from build123d import *

# Parameters (mm, degrees)
CROQUIS1_W                = 138
CROQUIS1_H                = 220
SALIENTE_EXTRUIR1_DEPTH   = 15
CORTAR_EXTRUIR1_DEPTH     = 76.5
CROQUIS3_R                = 4.25
CORTAR_EXTRUIR2_DEPTH     = 76.5
CROQUIS4_R                = 6.5
CORTAR_EXTRUIR3_DEPTH     = 8
CROQUIS5_W                = 12
CROQUIS5_H                = 220
CORTAR_EXTRUIR4_DEPTH     = 4
TALADRO_ROSCADO_M41_D     = 3.3
TALADRO_ROSCADO_M41_DEPTH = 8
TALADRO_ROSCADO_M41_TIP   = 0.991420021
CORTAR_EXTRUIR5_DEPTH     = 8
CHAFL_N1_SIZE             = 2


with BuildPart() as part:
    # Croquis1 → Saliente-Extruir1 (new body)
    with BuildSketch(Plane.XY):
        Rectangle(CROQUIS1_W, CROQUIS1_H)
    extrude(amount=SALIENTE_EXTRUIR1_DEPTH)

    # Croquis2 → Cortar-Extruir1 (cut)
    with BuildSketch(Plane.XY.offset(15)):
        with BuildLine():
            Line((-56, 122.891872251), (-56, 98))
            ThreePointArc((-56, 98), (-50, 92), (-44, 98))
            Line((-44, 98), (-44, 122.891872251))
            Line((-44, 122.891872251), (-56, 122.891872251))
        make_face()
        with BuildLine():
            Line((44, 116.909766475), (44, 98))
            ThreePointArc((44, 98), (50, 92), (56, 98))
            Line((56, 98), (56, 116.909766475))
            Line((56, 116.909766475), (44, 116.909766475))
        make_face()
        with BuildLine():
            Line((44, -98), (44, -115.830663504))
            Line((44, -115.830663504), (56, -115.830663504))
            Line((56, -115.830663504), (56, -98))
            ThreePointArc((56, -98), (50, -92), (44, -98))
        make_face()
        with BuildLine():
            Line((-56, -98), (-56, -115.886145335))
            Line((-56, -115.886145335), (-44, -115.886145335))
            Line((-44, -115.886145335), (-44, -98))
            ThreePointArc((-44, -98), (-50, -92), (-56, -98))
        make_face()
    extrude(amount=-CORTAR_EXTRUIR1_DEPTH, mode=Mode.SUBTRACT)

    # Croquis3 → Cortar-Extruir2 (cut)
    with BuildSketch(Plane.XY.offset(15)):
        with Locations((-61.5, 82.5)):
            Circle(CROQUIS3_R)
        with Locations((-61.5, 23.7)):
            Circle(CROQUIS3_R)
        with Locations((-61.5, -35.1)):
            Circle(CROQUIS3_R)
        with Locations((-34, -78.5)):
            Circle(CROQUIS3_R)
        with Locations((34, -78.5)):
            Circle(CROQUIS3_R)
        with Locations((61.5, -35.1)):
            Circle(CROQUIS3_R)
        with Locations((61.5, 23.7)):
            Circle(CROQUIS3_R)
        with Locations((61.5, 82.5)):
            Circle(CROQUIS3_R)
    extrude(amount=-CORTAR_EXTRUIR2_DEPTH, mode=Mode.SUBTRACT)

    # Croquis4 → Cortar-Extruir3 (cut)
    with BuildSketch(Plane.XY.offset(15)):
        with Locations((-61.5, 82.5)):
            Circle(CROQUIS4_R)
        with Locations((-61.5, 23.7)):
            Circle(CROQUIS4_R)
        with Locations((-61.5, -35.1)):
            Circle(CROQUIS4_R)
        with Locations((-34, -78.5)):
            Circle(CROQUIS4_R)
        with Locations((61.5, -35.1)):
            Circle(CROQUIS4_R)
        with Locations((61.5, 23.7)):
            Circle(CROQUIS4_R)
        with Locations((61.5, 82.5)):
            Circle(CROQUIS4_R)
        with Locations((34, -78.5)):
            Circle(CROQUIS4_R)
    extrude(amount=-CORTAR_EXTRUIR3_DEPTH, mode=Mode.SUBTRACT)

    # Croquis5 → Cortar-Extruir4 (cut)
    with BuildSketch(Plane.XY.offset(15)):
        Rectangle(CROQUIS5_W, CROQUIS5_H)
    extrude(amount=-CORTAR_EXTRUIR4_DEPTH, mode=Mode.SUBTRACT)

    # Taladro roscado M41
    with Locations(Plane.XY.offset(11)):
        with Locations((0, 104), (0, 76), (0, 14), (0, -14), (0, -76), (0, -104)):
            Hole(TALADRO_ROSCADO_M41_D / 2, depth=TALADRO_ROSCADO_M41_DEPTH)
            with Locations((0, 0, -(TALADRO_ROSCADO_M41_DEPTH + TALADRO_ROSCADO_M41_TIP / 2))):  # 118° drill point
                Cone(0, TALADRO_ROSCADO_M41_D / 2, TALADRO_ROSCADO_M41_TIP, mode=Mode.SUBTRACT)

    # Croquis8 → Cortar-Extruir5 (cut)
    with BuildSketch(Plane(origin=(0, 0, 0), x_dir=(-1, 0, 0), z_dir=(0, 0, -1))):
        with BuildLine():
            Line((30, -55.5), (-30, -55.5))
            ThreePointArc((-30, -55.5), (-34.242640687, -53.742640687), (-36, -49.5))
            Line((-36, -49.5), (-36, 66.5))
            ThreePointArc((-36, 66.5), (-34.242640687, 70.742640687), (-30, 72.5))
            Line((-30, 72.5), (30, 72.5))
            ThreePointArc((30, 72.5), (34.242640687, 70.742640687), (36, 66.5))
            Line((36, 66.5), (36, -49.5))
            ThreePointArc((36, -49.5), (34.242640687, -53.742640687), (30, -55.5))
        make_face()
    extrude(amount=-CORTAR_EXTRUIR5_DEPTH, mode=Mode.SUBTRACT)

    # Chaflán1
    chafl_n1_edges = [part.edges().sort_by_distance(p)[0] for p in [
        (34.242640687, 70.742640687, 0),
        (36, 8.5, 0),
        (34.242640687, -53.742640687, 0),
        (0, -55.5, 0),
        (-34.242640687, -53.742640687, 0),
        (-36, 8.5, 0),
        (-34.242640687, 70.742640687, 0),
        (0, 72.5, 0),
    ]]
    chamfer(chafl_n1_edges, length=CHAFL_N1_SIZE)


solid = part.part
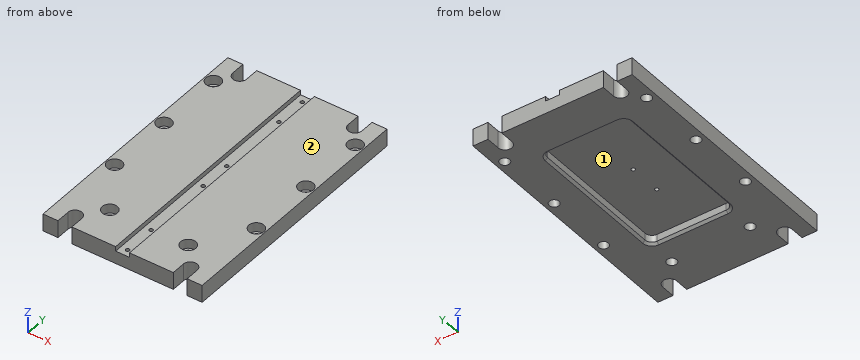
Geometry: final body of the model. Coordinates: model frame, mm. Face numbers are marked on the shaded views. Round coordinates to 2 decimals unless told otherwise and drop trailing zeros. Loops run counter-clockwise (first coordinate to the right, second up) from the corner with the lowest first, then second, coordinate; pieces in that order, holes last.
Q1. Section A-A on x = -61.5. Return loops of the section in (y, z).
Q2. Pull-direction query (X, two-part tool) for the marked faces 1 and 2; classes: released by +X, released by -X, zero draft, split by the parting line, or undercut.
Q3. Pin query (flat end, axial travel): P1, Ø10.5, axis at x = -61.5, y = 82.5, coming from the +Z side; P2, Ø21.5, axis at x = 11.5, y = 0.5, coming from the -Z side; P3, Ø4, axis at x = 0, y = 104, coming from the +Z side. Return the tip coordinate at first contact, or that it passes through.
Q4. Section C-C on y = 36. Return loops of the section in (x, z).
Q5. Section D-D on y = -35.1. State how many separate pieces and enclosed holes the cut face has, plus the area to 4 significant figures.
Q6. Material intervals for L1, parallel to Y at x = -61.5, z = 3.5; L2, parallel to Y at x = 28.5, z = 3; L3, parallel to X at y = 72.5, z = 12, sorted ascending.
Q7. Section B-B on y = 82.5. Return loops of the section in (x, z), plus the area to 4 significant figures.
Evaluation:
1. outline: (-110, 0) - (-39.35, 0) - (-39.35, 7) - (-41.6, 7) - (-41.6, 15) - (-110, 15) - close; (-30.85, 0) - (19.45, 0) - (19.45, 7) - (17.2, 7) - (17.2, 15) - (-28.6, 15) - (-28.6, 7) - (-30.85, 7) - close; (27.95, 0) - (78.25, 0) - (78.25, 7) - (76, 7) - (76, 15) - (30.2, 15) - (30.2, 7) - (27.95, 7) - close; (86.75, 0) - (110, 0) - (110, 15) - (89, 15) - (89, 7) - (86.75, 7) - close
2. face 1: undercut
2. face 2: zero draft
3. P1: stops at z = 7
3. P2: stops at z = 8
3. P3: stops at z = 11
4. outline: (-69, 0) - (-38, 0) - (-36, 2) - (-36, 8) - (36, 8) - (36, 2) - (38, 0) - (69, 0) - (69, 15) - (6, 15) - (6, 11) - (-6, 11) - (-6, 15) - (-69, 15) - close
5. separate pieces: 3
5. enclosed holes: 0
5. area: 1,115 mm2
6. L1: y = -110 to -39.35, -30.85 to 19.45, 27.95 to 78.25, 86.75 to 110
6. L2: y = -110 to -55.5, 72.5 to 110
6. L3: x = -69 to -6, 6 to 69
7. outline: (-69, 0) - (-65.75, 0) - (-65.75, 7) - (-68, 7) - (-68, 15) - (-69, 15) - close; (-57.25, 0) - (57.25, 0) - (57.25, 7) - (55, 7) - (55, 15) - (6, 15) - (6, 11) - (-6, 11) - (-6, 15) - (-55, 15) - (-55, 7) - (-57.25, 7) - close; (65.75, 0) - (69, 0) - (69, 15) - (68, 15) - (68, 7) - (65.75, 7) - close
7. area: 1,695 mm2
